Geometry: final body of the model. Coordinates: model frame, mm. A direction names the side the tool comes from. Coordinates: 2 decimals unless noted, no trailing zeros. Loops run counter-clockwise (first coordinate to the right, second up) from the corner with the lowest first, then second, coordinate; pieces in that order, holes last. Notation, with made-up numbers: (-38, 51) -> (3, 51) arc R12 cw to (3, 68) -> close; hole circle Ø1 at (38, 56.5). An arc over 180 degrees is marked (long way). One line per item, written item: value. Start each with the question number.
from build123d import *

# Parameters (mm, degrees)
F1_DEPTH      = 39
F1_DEPTH_BACK = 15
F2_W          = 23.6637403975
F2_H          = 12
F3_DEPTH      = 15
F4_D          = 3.2
F5_W          = 7.9318701987
F5_H          = 11
F6_DEPTH      = 6
F9_DEPTH      = 6.5
F10_DEPTH     = 12
F11_W         = 6
F11_H         = 35
F12_DEPTH     = 7
F13_W         = 6
F13_H         = 35
F14_DEPTH     = 7
F15_R         = 5
F16_R         = 5
F18_D         = 3


with BuildPart() as f1:
    # F0 (on Top) → F1 (new body, two sides)
    with BuildSketch(Plane.XY) as f1_sk:
        Polygon((-11.8318701987, 6), (-11.8318701987, 0), (-11.8318701987, -2.6806737598), (-11.8318701987, -12), (-3.9, -12), (-3.9, 0), (0, 0), (3.9, 0), (3.9, -12), (11.8318701987, -12), (11.8318701987, -2.6806737598), (11.8318701987, 0), (11.8318701987, 6), (0, 6), align=None)
    extrude(amount=F1_DEPTH)
    extrude(f1_sk.sketch, amount=-F1_DEPTH_BACK)

    # F2 (on Top) → F3 (join, through all)
    with BuildSketch(Plane.XY):
        with Locations((0, -6)):
            Rectangle(F2_W, F2_H)
    extrude(amount=-F3_DEPTH)

    # F4 (through all)
    with Locations(Plane.XY):
        with Locations((0, -3.5)):
            Hole(F4_D / 2)

    # F5 (on face) → F6 (cut)
    with BuildSketch(Plane.XZ.offset(12)):
        with Locations((7.8659350994, 5.5)):
            Rectangle(F5_W, F5_H)
        with Locations((-7.8659350994, 5.5)):
            Rectangle(F5_W, F5_H)
    extrude(amount=-F6_DEPTH, mode=Mode.SUBTRACT)

    # F8 (on offset) → F9 (cut)
    with BuildSketch(Plane.XY.offset(36)):
        with BuildLine():
            Line((8.0307415794, -12), (8.0307415794, -3.5038522084))
            ThreePointArc((8.0307415794, -3.5038522084), (0.0307415794, 4.4961477916), (-7.9692584206, -3.5038522084))
            Line((-7.9692584206, -3.5038522084), (-7.9692584206, -12))
            Line((-7.9692584206, -12), (3.9, -12))
            Line((3.9, -12), (8.0307415794, -12))
        make_face()
    extrude(amount=-F9_DEPTH, mode=Mode.SUBTRACT)

    # F10 (add, through all): a face of the model
    f10_faces = [f1.faces().sort_by_distance(p)[0] for p in [
        (0, 0, 37.5),
    ]]
    extrude(f10_faces, amount=F10_DEPTH)

    # F11 (on face) → F12 (join)
    with BuildSketch(Plane(origin=(-11.8318701987, 0, 0), x_dir=(0, -1, 0), z_dir=(-1, 0, 0))):
        with Locations((-3, 21.5)):
            Rectangle(F11_W, F11_H)
    extrude(amount=F12_DEPTH)

    # F13 (on face) → F14 (join)
    with BuildSketch(Plane.YZ.offset(11.8318701987)):
        with Locations((3, 21.5)):
            Rectangle(F13_W, F13_H)
    extrude(amount=F14_DEPTH)

    # F15
    f15_edges = [f1.edges().sort_by_distance(p)[0] for p in [
        (-18.83187, 3, 39),
        (-18.83187, 3, 4),
        (18.83187, 3, 4),
        (18.83187, 3, 39),
        (-11.83187, -6, 39),
        (11.83187, -6, 39),
    ]]
    fillet(f15_edges, radius=F15_R)

    # F16
    f16_edges = [f1.edges().sort_by_distance(p)[0] for p in [
        (-11.83187, -3, -15),
        (0, -12, -15),
        (11.83187, -3, -15),
        (0, 6, -15),
    ]]
    fillet(f16_edges, radius=F16_R)

    # F18 (through all)
    with Locations(Plane(origin=(0, 6, 0), x_dir=(-1, 0, 0), z_dir=(0, 1, 0))):
        with Locations((-15.3318701987, 32.3067344725), (-15.3318701987, 12.3429447412), (15.3318701987, 12.3429447412), (15.3318701987, 32.3067344725)):
            Hole(F18_D / 2)


solid = f1.part
1. Pin query (flat end, axial travel): pin 1 Ø10 at (x, y) = (-8.5, -2) entering from -Z; pin 2 Ø5 at (y, z) = (-9.5, 32.5) entering from -X; pin 3 Ø2 at (y, z) = (-5.5, 32.5) entering from +X; pin 4 Ø8.5 at (x, z) = (6, 6) entering from -Y. Return the tip coordinate at first contact, or that it passes through.
2. Section D-D on y = -4.25. Return the cut outline in (x, z), plus the area to 3 significant figures.
3. Set-up query: faces 5 (the face through (-8, -9, 11)), 6 (the face through (-2, -3, -15)), 7 (the face through (-3.9, -6, 18)). Return all of +Z, -Z, +X, -X, +Y, -Y with unobstructed straight access to the full face (end or side cutting, diameter ignored); none if empty.
4. Line query: L1, parallel to Z at x = 5.5, y = -0.75; L2, parallel to X at y = -7.5, z = 23.5; L3, parallel to X at y = -7.25, z = 32. Output: solid intervals per line, ascending. Write a range as [from, to].
5. Section B-B on z = 3. Return the cut outline in (x, y).
6. Section C-C on x = 15.5. Return the cut outline in (y, z).
7. Section A-A on x = 0. Return the cut outline in (y, z), plus the area to 3 significant figures.
8. Draft query along Y for faces 1 (the face through (0, -10, -14)), 2 (the face through (0.208, -1.914, -7.605)), 3 (the face through (0, -7, 0)), 4 (the face through (0, 4, -14)). Return one class per face: released by +Y, released by -Y, zero draft, split by the parting line, or undercut.
Checks:
1. pin 1: z = -15
1. pin 2: x = -11.83
1. pin 3: x = 11.83
1. pin 4: y = -6
2. outline: (-11.83, -10) arc R5 ccw to (-6.83, -15) -> (-1.41, -15) -> (-1.41, 0) -> (-3.9, 0) -> (-3.9, 29.5) -> (-7.97, 29.5) -> (-7.97, 36) -> (8.03, 36) -> (8.03, 29.5) -> (3.9, 29.5) -> (3.9, 0) -> (1.41, 0) -> (1.41, -15) -> (6.83, -15) arc R5 ccw to (11.83, -10) -> (11.83, 34) arc R5 ccw to (6.83, 39) -> (-6.83, 39) arc R5 ccw to (-11.83, 34) -> close
2. area: 880 mm²
3. face 5: +X, -X, -Y
3. face 6: -Z, +X, -X, +Y, -Y
3. face 7: -Y
4. L1: [-15, 29.5], [36, 39]
4. L2: [-11.83, -3.9], [3.9, 11.83]
4. L3: [-11.83, -7.97], [8.03, 11.83]
5. outline: (-11.83, -6) -> (-3.9, -6) -> (-3.9, 0) -> (3.9, 0) -> (3.9, -6) -> (11.83, -6) -> (11.83, 6) -> (-11.83, 6) -> close
6. outline: (0, 4.29) -> (6, 4.29) -> (6, 10.85) -> (0, 10.85) -> close; (0, 13.83) -> (6, 13.83) -> (6, 30.82) -> (0, 30.82) -> close; (0, 33.8) -> (6, 33.8) -> (6, 38.71) -> (0, 38.71) -> close
7. outline: (-12, -10) arc R5 ccw to (-7, -15) -> (-5.1, -15) -> (-5.1, 0) -> (-12, 0) -> close; (-12, 36) -> (4.5, 36) -> (4.5, 29.5) -> (0, 29.5) -> (0, 0) -> (-1.9, 0) -> (-1.9, -15) -> (1, -15) arc R5 ccw to (6, -10) -> (6, 39) -> (-12, 39) -> close
7. area: 452 mm²
8. face 1: released by -Y
8. face 2: undercut
8. face 3: zero draft
8. face 4: released by +Y
